Build history of the part. All positions in model axes, mm. Coordinates: 2 decimals unless noted, no trailing zeros. Write each loop counter-clockwise with the first axis right and the second up, starting at its lowest first coordinate (ties: lowest second). Pieces come first, ordered by that corner, then holes. Notation, with made-up numbers: M 28,69.25 L 39,69.25 A22 ccw 39,84.25 Z; hole C 31.25,29.5 d8. An arc over 180 degrees is marked long. Use CSV: the item, a comma, the result in double quotes. Start each with the question number.
```python
from build123d import *

# Parameters (mm, degrees)
F0_R     = 1.6
F1_DEPTH = 3.175


# Not quite as in the source:
# - a length typed as a fraction of an inch, garbled in the dataset ("3 / 203.2 mm" for 3/8 in), is restored


with BuildPart() as f1:
    # F0 (on Front) → F1 (new body)
    with BuildSketch(Plane.XZ):
        with BuildLine():
            Line((143.65, 0), (6.35, 0))
            ThreePointArc((6.35, 0), (1.8598719395, -1.8598719395), (0, -6.35))
            Line((0, -6.35), (0, -103.65))
            ThreePointArc((0, -103.65), (1.8598719395, -108.1401280605), (6.35, -110))
            Line((6.35, -110), (143.65, -110))
            ThreePointArc((143.65, -110), (148.1401280605, -108.1401280605), (150, -103.65))
            Line((150, -103.65), (150, -6.35))
            ThreePointArc((150, -6.35), (148.1401280605, -1.8598719395), (143.65, 0))
        make_face()
        with Locations((5, -105)):
            Circle(F0_R, mode=Mode.SUBTRACT)
        with Locations((15, -105)):
            Circle(F0_R, mode=Mode.SUBTRACT)
        with Locations((25, -105)):
            Circle(F0_R, mode=Mode.SUBTRACT)
        with Locations((35, -105)):
            Circle(F0_R, mode=Mode.SUBTRACT)
        with Locations((5, -95)):
            Circle(F0_R, mode=Mode.SUBTRACT)
        with Locations((15, -95)):
            Circle(F0_R, mode=Mode.SUBTRACT)
        with Locations((5, -85)):
            Circle(F0_R, mode=Mode.SUBTRACT)
        with Locations((25, -95)):
            Circle(F0_R, mode=Mode.SUBTRACT)
        with Locations((25, -85)):
            Circle(F0_R, mode=Mode.SUBTRACT)
        with Locations((45, -105)):
            Circle(F0_R, mode=Mode.SUBTRACT)
        with Locations((55, -105)):
            Circle(F0_R, mode=Mode.SUBTRACT)
        with Locations((65, -105)):
            Circle(F0_R, mode=Mode.SUBTRACT)
        with Locations((5, -75)):
            Circle(F0_R, mode=Mode.SUBTRACT)
        with Locations((31.077, -77.1057)):
            Circle(F0_R, mode=Mode.SUBTRACT)
        with Locations((5, -65)):
            Circle(F0_R, mode=Mode.SUBTRACT)
        with BuildLine():
            ThreePointArc((10, -24.0538), (11.1159231637, -21.3597231637), (13.81, -20.2438))
            Line((13.81, -20.2438), (16.19, -20.2438))
            ThreePointArc((16.19, -20.2438), (18.8840768363, -21.3597231637), (20, -24.0538))
            Line((20, -24.0538), (20, -85.9536))
            ThreePointArc((20, -85.9536), (18.8840768363, -88.6476768363), (16.19, -89.7636))
            Line((16.19, -89.7636), (13.81, -89.7636))
            ThreePointArc((13.81, -89.7636), (11.1159231637, -88.6476768363), (10, -85.9536))
            Line((10, -85.9536), (10, -24.0538))
        make_face(mode=Mode.SUBTRACT)
        with Locations((24.492, -65)):
            Circle(F0_R, mode=Mode.SUBTRACT)
        with Locations((75, -105)):
            Circle(F0_R, mode=Mode.SUBTRACT)
        with Locations((85, -105)):
            Circle(F0_R, mode=Mode.SUBTRACT)
        with Locations((95, -105)):
            Circle(F0_R, mode=Mode.SUBTRACT)
        with Locations((105, -105)):
            Circle(F0_R, mode=Mode.SUBTRACT)
        with Locations((75, -95.9955)):
            Circle(F0_R, mode=Mode.SUBTRACT)
        with Locations((115, -105)):
            Circle(F0_R, mode=Mode.SUBTRACT)
        with Locations((125, -105)):
            Circle(F0_R, mode=Mode.SUBTRACT)
        with Locations((135, -105)):
            Circle(F0_R, mode=Mode.SUBTRACT)
        with Locations((145, -105)):
            Circle(F0_R, mode=Mode.SUBTRACT)
        with Locations((125, -95)):
            Circle(F0_R, mode=Mode.SUBTRACT)
        with Locations((125, -85)):
            Circle(F0_R, mode=Mode.SUBTRACT)
        with Locations((135, -95)):
            Circle(F0_R, mode=Mode.SUBTRACT)
        with Locations((145, -95)):
            Circle(F0_R, mode=Mode.SUBTRACT)
        with Locations((145, -85)):
            Circle(F0_R, mode=Mode.SUBTRACT)
        with BuildLine():
            Line((49.6062, -83.4136), (49.6062, -26.5938))
            ThreePointArc((49.6062, -26.5938), (51.4660719395, -22.1036719395), (55.9562, -20.2438))
            Line((55.9562, -20.2438), (94.0562, -20.2438))
            ThreePointArc((94.0562, -20.2438), (98.5463280605, -22.1036719395), (100.4062, -26.5938))
            Line((100.4062, -26.5938), (100.4062, -83.4136))
            ThreePointArc((100.4062, -83.4136), (98.5463280605, -87.9037280605), (94.0562, -89.7636))
            Line((94.0562, -89.7636), (55.9562, -89.7636))
            ThreePointArc((55.9562, -89.7636), (51.4660719395, -87.9037280605), (49.6062, -83.4136))
        make_face(mode=Mode.SUBTRACT)
        with Locations((111.077, -55.0037)):
            Circle(F0_R, mode=Mode.SUBTRACT)
        with Locations((125, -75)):
            Circle(F0_R, mode=Mode.SUBTRACT)
        with Locations((145, -75)):
            Circle(F0_R, mode=Mode.SUBTRACT)
        with Locations((125, -65)):
            Circle(F0_R, mode=Mode.SUBTRACT)
        with Locations((145, -65)):
            Circle(F0_R, mode=Mode.SUBTRACT)
        with BuildLine():
            ThreePointArc((130, -24.0538), (131.1159231637, -21.3597231637), (133.81, -20.2438))
            Line((133.81, -20.2438), (136.19, -20.2438))
            ThreePointArc((136.19, -20.2438), (138.8840768363, -21.3597231637), (140, -24.0538))
            Line((140, -24.0538), (140, -85.9536))
            ThreePointArc((140, -85.9536), (138.8840768363, -88.6476768363), (136.19, -89.7636))
            Line((136.19, -89.7636), (133.81, -89.7636))
            ThreePointArc((133.81, -89.7636), (131.1159231637, -88.6476768363), (130, -85.9536))
            Line((130, -85.9536), (130, -24.0538))
        make_face(mode=Mode.SUBTRACT)
        with Locations((5, -55)):
            Circle(F0_R, mode=Mode.SUBTRACT)
        with Locations((5, -45)):
            Circle(F0_R, mode=Mode.SUBTRACT)
        with Locations((24.492, -55)):
            Circle(F0_R, mode=Mode.SUBTRACT)
        with Locations((24.492, -45)):
            Circle(F0_R, mode=Mode.SUBTRACT)
        with Locations((5, -35)):
            Circle(F0_R, mode=Mode.SUBTRACT)
        with Locations((31.077, -32.9057)):
            Circle(F0_R, mode=Mode.SUBTRACT)
        with Locations((5, -25)):
            Circle(F0_R, mode=Mode.SUBTRACT)
        with Locations((5, -15)):
            Circle(F0_R, mode=Mode.SUBTRACT)
        with Locations((15, -15)):
            Circle(F0_R, mode=Mode.SUBTRACT)
        with Locations((24.492, -25)):
            Circle(F0_R, mode=Mode.SUBTRACT)
        with Locations((25, -15)):
            Circle(F0_R, mode=Mode.SUBTRACT)
        with Locations((5, -5)):
            Circle(F0_R, mode=Mode.SUBTRACT)
        with Locations((15, -5)):
            Circle(F0_R, mode=Mode.SUBTRACT)
        with Locations((25, -5)):
            Circle(F0_R, mode=Mode.SUBTRACT)
        with Locations((35, -5)):
            Circle(F0_R, mode=Mode.SUBTRACT)
        with Locations((52.9082, -15.9955)):
            Circle(F0_R, mode=Mode.SUBTRACT)
        with Locations((45, -5)):
            Circle(F0_R, mode=Mode.SUBTRACT)
        with Locations((55, -5)):
            Circle(F0_R, mode=Mode.SUBTRACT)
        with Locations((65, -5)):
            Circle(F0_R, mode=Mode.SUBTRACT)
        with Locations((125, -55)):
            Circle(F0_R, mode=Mode.SUBTRACT)
        with Locations((125, -45)):
            Circle(F0_R, mode=Mode.SUBTRACT)
        with Locations((145, -55)):
            Circle(F0_R, mode=Mode.SUBTRACT)
        with Locations((145, -45)):
            Circle(F0_R, mode=Mode.SUBTRACT)
        with Locations((125, -35)):
            Circle(F0_R, mode=Mode.SUBTRACT)
        with Locations((145, -35)):
            Circle(F0_R, mode=Mode.SUBTRACT)
        with Locations((97.1082, -15.9955)):
            Circle(F0_R, mode=Mode.SUBTRACT)
        with Locations((75, -5)):
            Circle(F0_R, mode=Mode.SUBTRACT)
        with Locations((85, -5)):
            Circle(F0_R, mode=Mode.SUBTRACT)
        with Locations((95, -5)):
            Circle(F0_R, mode=Mode.SUBTRACT)
        with Locations((105, -5)):
            Circle(F0_R, mode=Mode.SUBTRACT)
        with Locations((125, -25)):
            Circle(F0_R, mode=Mode.SUBTRACT)
        with Locations((125, -15)):
            Circle(F0_R, mode=Mode.SUBTRACT)
        with Locations((145, -25)):
            Circle(F0_R, mode=Mode.SUBTRACT)
        with Locations((135, -15)):
            Circle(F0_R, mode=Mode.SUBTRACT)
        with Locations((145, -15)):
            Circle(F0_R, mode=Mode.SUBTRACT)
        with Locations((115, -5)):
            Circle(F0_R, mode=Mode.SUBTRACT)
        with Locations((125, -5)):
            Circle(F0_R, mode=Mode.SUBTRACT)
        with Locations((135, -5)):
            Circle(F0_R, mode=Mode.SUBTRACT)
        with Locations((145, -5)):
            Circle(F0_R, mode=Mode.SUBTRACT)
    extrude(amount=F1_DEPTH)


solid = f1.part
```
1. Slice it at C-C (y = -0.65). Count the separate pieces of the cut face and the enclosed holes in it, and give its area (3 significant figures).
2. Slice it at A-A (z = -50). List the corners of the cut face in (x, y) (3 decimals), and give its area (3 significant figures).
3. Slice it at B-B (x = 105). List the corners of the cut face in (y, z) (3 decimals), and give its area (3 significant figures).
4. Drill centre lines: line 1 along Z through (x, y) = (135, -1.15); line 2 along Z through (x, y) = (75, -2.4); line 3 along X through (y, z) = (-1.25, -41). Where is each one in solid material? Low to high. Write a range as from..to.
Established:
1,separate pieces,"1"
1,enclosed holes,"77"
1,area,"11,000 mm2"
2,outline,"M 0,-3.175 L 10,-3.175 L 10,0 L 0,0 Z; M 20,-3.175 L 49.606,-3.175 L 49.606,0 L 20,0 Z; M 100.406,-3.175 L 130,-3.175 L 130,0 L 100.406,0 Z; M 140,-3.175 L 150,-3.175 L 150,0 L 140,0 Z"
2,area,"251 mm2"
3,outline,"M -3.175,-110 L 0,-110 L 0,-106.6 L -3.175,-106.6 Z; M -3.175,-103.4 L 0,-103.4 L 0,-6.6 L -3.175,-6.6 Z; M -3.175,-3.4 L 0,-3.4 L 0,0 L -3.175,0 Z"
3,area,"329 mm2"
4,line 1,"z = -110..-106.6, -103.4..-96.6, -93.4..-89.76, -20.24..-16.6, -13.4..-6.6, -3.4..0"
4,line 2,"z = -110..-106.6, -103.4..-97.6, -94.4..-89.76, -20.24..-6.6, -3.4..0"
4,line 3,"x = 0..10, 20..49.61, 100.41..130, 140..150"
